from build123d import *

# Parameters (mm, degrees)
SKETCH1_R                                         = 11
SKETCH1_R_2                                       = 5
SKETCH1_R_3                                       = 3.50012
BODY_DEPTH                                        = 3.175
CSK_FOR_M2_5_FLAT_HEAD_MACHINE_SCREW1_D           = 2.9
CSK_FOR_M2_5_FLAT_HEAD_MACHINE_SCREW1_CSINK_D     = 5.5
CSK_FOR_M2_5_FLAT_HEAD_MACHINE_SCREW1_CSINK_ANGLE = 90
FILLET1_R                                         = 5
F_10_32_TAPPED_HOLE2_D                            = 4.0386
F_10_32_TAPPED_HOLE2_DEPTH                        = 12.03
F_10_32_TAPPED_HOLE2_TIP                          = 1.213317848
F_6_32_TAPPED_HOLE1_D                             = 2.7051
F_6_32_TAPPED_HOLE1_DEPTH                         = 9.39
F_6_32_TAPPED_HOLE1_TIP                           = 0.81269403
SKETCH1_3_R                                       = 5
SKETCH1_3_R_2                                     = 3.50012
MOTOR_COLLAR_RECESS_DEPTH                         = 1.82626


with BuildPart() as part:
    # Sketch1 → Body (new body)
    # profile 1 of 7: a face of its own
    with BuildSketch(Plane.XY):
        with BuildLine():
            ThreePointArc((22, 0), (0, 22), (-22, 0))
            ThreePointArc((-22, 0), (-21.570998032, -4.323429644), (-20.300723283, -8.478244759))
            ThreePointArc((-20.300723283, -8.478244759), (-20.230414586, -8.644670364), (-20.158741556, -8.810512975))
            ThreePointArc((-20.158741556, -8.810512975), (-12.045096815, -18.409661668), (0, -22))
            ThreePointArc((0, -22), (15.556349186, -15.556349186), (22, 0))
        make_face()
    # profile 2 of 7: a face of its own
    with BuildSketch(Plane.XY):
        with BuildLine():
            Line((-19.557278205, -22), (0, -22))
            ThreePointArc((0, -22), (-12.045096815, -18.409661668), (-20.158741556, -8.810512975))
            Line((-20.158741556, -8.810512975), (-20.159744108, -8.824772966))
            ThreePointArc((-20.159744108, -8.824772966), (-19.094742513, -12.488878324), (-18.735496202, -16.28767268))
            ThreePointArc((-18.735496202, -16.28767268), (-18.94199382, -19.173240608), (-19.557278205, -22))
        make_face()
    # profile 3 of 7: a face of its own
    with BuildSketch(Plane.XY):
        with BuildLine():
            ThreePointArc((-18.735496202, -16.28767268), (-19.094742513, -12.488878324), (-20.159744108, -8.824772966))
            Line((-20.159744108, -8.824772966), (-21.086031744, -22))
            Line((-21.086031744, -22), (-19.557278205, -22))
            ThreePointArc((-19.557278205, -22), (-18.94199382, -19.173240608), (-18.735496202, -16.28767268))
        make_face()
    # profile 4 of 7: a face of its own
    with BuildSketch(Plane.XY):
        with BuildLine():
            ThreePointArc((-20.300723283, -8.478244759), (-21.570998032, -4.323429644), (-22, 0))
            Line((-22, 0), (-25.571764484, -1.110960087))
            ThreePointArc((-25.571764484, -1.110960087), (-22.519299729, -4.496293084), (-20.300723283, -8.478244759))
        make_face()
    # profile 5 of 7: a face of its own
    with BuildSketch(Plane.XY):
        with BuildLine():
            ThreePointArc((-20.300723283, -8.478244759), (-22.519299729, -4.496293084), (-25.571764484, -1.110960087))
            Line((-25.571764484, -1.110960087), (-39, -5.28767268))
            ThreePointArc((-39, -5.28767268), (-31.221825407, -8.509498087), (-28, -16.28767268))
            ThreePointArc((-28, -16.28767268), (-28.407421205, -19.253692652), (-29.59950445, -22))
            Line((-29.59950445, -22), (-21.086031744, -22))
            Line((-21.086031744, -22), (-20.159744108, -8.824772966))
            ThreePointArc((-20.159744108, -8.824772966), (-20.22943401, -8.651183524), (-20.300723283, -8.478244759))
        make_face()
    # profile 6 of 7: a face of its own
    with BuildSketch(Plane.XY):
        with Locations((-39, -16.28767268)):
            Circle(SKETCH1_R)
        with Locations((-39, -16.28767268)):
            Circle(SKETCH1_R_2, mode=Mode.SUBTRACT)
    # profile 7 of 7: a face of its own
    with BuildSketch(Plane.XY):
        with Locations((-39, -16.28767268)):
            Circle(SKETCH1_R_2)
        with Locations((-39, -16.28767268)):
            Circle(SKETCH1_R_3, mode=Mode.SUBTRACT)
    extrude(amount=BODY_DEPTH)

    # CSK for M2.5 Flat Head Machine Screw1 (through all)
    with Locations(Plane(origin=(-39, -9.28767268, 3.175), x_dir=(1, 0, 0), z_dir=(0, 0, 1))):
        with Locations((0, 0), (-6.062177826, -10.5), (6.062177826, -10.5)):
            CounterSinkHole(CSK_FOR_M2_5_FLAT_HEAD_MACHINE_SCREW1_D / 2, CSK_FOR_M2_5_FLAT_HEAD_MACHINE_SCREW1_CSINK_D / 2, counter_sink_angle=CSK_FOR_M2_5_FLAT_HEAD_MACHINE_SCREW1_CSINK_ANGLE)

    # Fillet1
    fillet1_edges = [part.edges().sort_by_distance(p)[0] for p in [
        (-29.59950445, -22, 1.5875),
        (-39, -5.28767268, 1.5875),
        (-22, 0, 1.5875),
    ]]
    fillet(fillet1_edges, radius=FILLET1_R)

    # 10-32 Tapped Hole2
    with Locations(Plane.XY.offset(3.175)):
        with Locations((0, 0)):
            Hole(F_10_32_TAPPED_HOLE2_D / 2, depth=F_10_32_TAPPED_HOLE2_DEPTH)
            with Locations((0, 0, -(F_10_32_TAPPED_HOLE2_DEPTH + F_10_32_TAPPED_HOLE2_TIP / 2))):  # 118° drill point
                Cone(0, F_10_32_TAPPED_HOLE2_D / 2, F_10_32_TAPPED_HOLE2_TIP, mode=Mode.SUBTRACT)

    # 6-32 Tapped Hole1
    with Locations(Plane(origin=(-8.660254038, 5, 0), x_dir=(-1, 0, 0), z_dir=(0, 0, -1))):
        with Locations((0, 0), (-17.320508076, 0), (-8.660254038, -15)):
            Hole(F_6_32_TAPPED_HOLE1_D / 2, depth=F_6_32_TAPPED_HOLE1_DEPTH)
            with Locations((0, 0, -(F_6_32_TAPPED_HOLE1_DEPTH + F_6_32_TAPPED_HOLE1_TIP / 2))):  # 118° drill point
                Cone(0, F_6_32_TAPPED_HOLE1_D / 2, F_6_32_TAPPED_HOLE1_TIP, mode=Mode.SUBTRACT)

    # Sketch1_3 → Motor Collar Recess (cut)
    with BuildSketch(Plane.XY):
        with Locations((-39, -16.28767268)):
            Circle(SKETCH1_3_R)
        with Locations((-39, -16.28767268)):
            Circle(SKETCH1_3_R_2, mode=Mode.SUBTRACT)
    extrude(amount=MOTOR_COLLAR_RECESS_DEPTH, mode=Mode.SUBTRACT)


solid = part.part
Verification items for the finished model (mm, model axes). A direction names the side the tool comes from. Coordinates: 2 decimals unless noted, no trailing zeros. Order: outer loops, then holes, each group sorted by start corner. A loop starts at its lowest first (then second) coordinate and runs counter-clockwise, first axis right, second up. Notation, with made-up numbers: M 36.25,35 L 74.25,35 A13 ccw 74.25,58 Z; hole C -4,74.25 d8. An arc over 180 degrees is marked long. One line per item, written item: value. Start each with the question number.
Item 1: Sectioned sample at D-D on y = 16. Record the cut outline in (x, z) (3 decimals).
Item 2: Sectioned sample at C-C on y = 5. Record the cut outline in (x, z) (3 decimals), then the cut area to 3 significant figures.
Item 3: Depth check by flat-ended pin: P1, Ø4, axis at x = -45.06, y = -19.79, coming from the +Z side; P2, Ø1, axis at x = 5.5, z = 2, coming from the -Y side; P3, Ø1, axis at x = -10.5, z = 2, coming from the -Y side. Enter the tip coordinate at first touch or a pass-through.
Item 4: Access from +Z, -Z, +X, -X, +Y, -Y to the whole of each face (thin tool, end or side, straight path). Record for faces 5 (the flat face through (-14, -22, 2)), 6 (the cylindrical face through (-43.995, -16.068, 0.9)), 7 (the cylindrical face through (-35.66, -15.24, 2.49)).
Item 5: Mould release check, pull along Y, two halves, no side actions. Record for faces 1 (the cylindrical face through (-49.06, -20.74, 1.57)), 2 (the flat face through (-37, -20, 1.826)), 3 (the flat face through (-7, -2, 3.175)), 4 (the cylindrical face through (-29.12, -22.42, 1.61)): pulls with the +Y half, pulls with the -Y half, needs draft (parallel to the pull), parting line crosses it, or undercut.
Item 6: Sectioned sample at B-B on z = 2.5. Give the number of separate pieces and of enclosed holes in the cut face, then the cut area to 3 significant figures.
Item 7: Sectioned sample at A-A on x = 9. Record the cut outline in (y, z) (3 decimals).
Item 8: Thickness scan on probe 1 along Y at (x, z) = (-39, 0.5); probe 2 along Y at (x, z) = (-39, 2.3); probe 3 along Y at (x, z) = (-47, 2.7). Record the ranges inside material, lowest first.
Calculated:
1. outline: M -15.1,0 L 15.1,0 L 15.1,3.175 L -15.1,3.175 Z
2. outline: M -21.424,0 L -10.013,0 L -10.013,3.175 L -21.424,3.175 Z; M -7.308,0 L 7.308,0 L 7.308,3.175 L -7.308,3.175 Z; M 10.013,0 L 21.424,0 L 21.424,3.175 L 10.013,3.175 Z
2. area: 119 mm^2
3. P1: z = 2.43
3. P2: y = -21.42
3. P3: y = -22
4. face 5: +Z, -Z, +X, -Y
4. face 6: -Z
4. face 7: +Z, -Z
5. face 1: parting line crosses it
5. face 2: undercut
5. face 3: needs draft
5. face 4: pulls with the -Y half
6. separate pieces: 1
6. enclosed holes: 9
6. area: 2,070 mm^2
7. outline: M -20.075,0 L 3.691,0 L 3.691,3.175 L -20.075,3.175 Z; M 6.309,0 L 20.075,0 L 20.075,3.175 L 6.309,3.175 Z
8. probe 1: -27.29 to -21.29, -11.29 to -10.74, -7.84 to -5.24
8. probe 2: -27.29 to -19.79, -12.79 to -11.16, -7.41 to -5.24
8. probe 3: -23.84 to -20.98, -18.6 to -8.74
